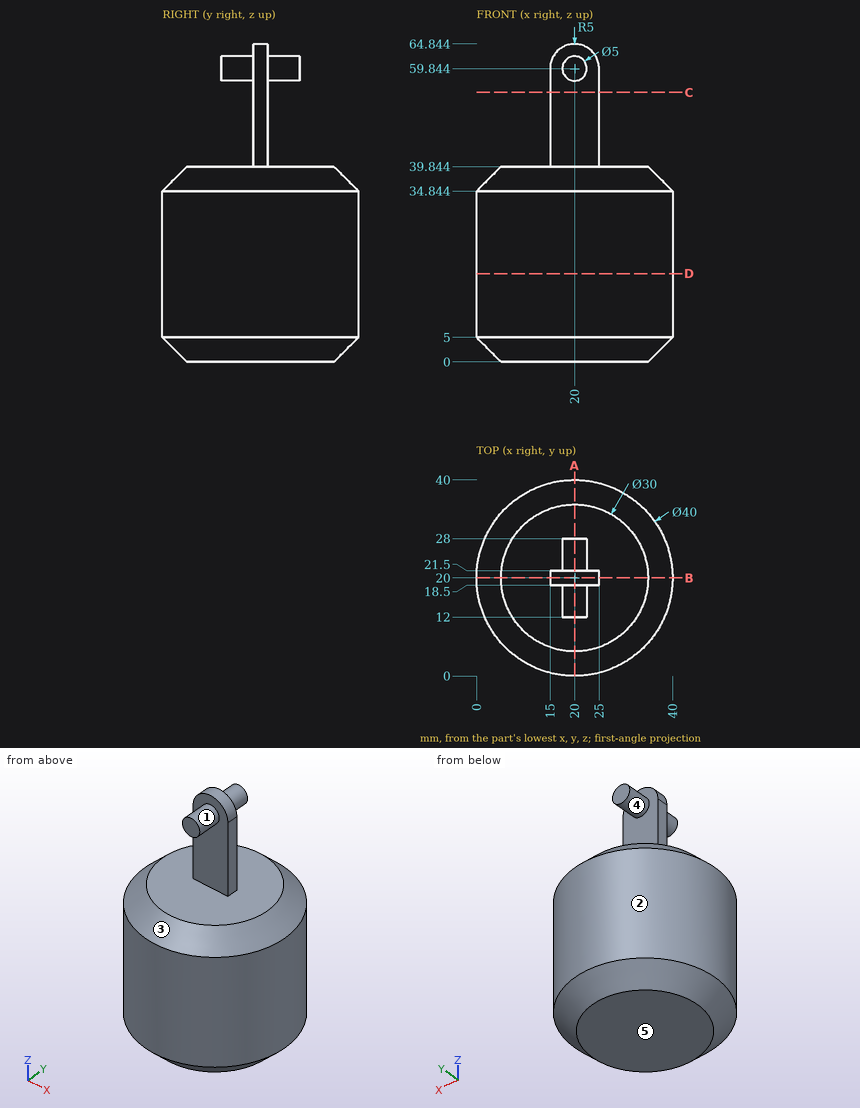
Study the drawing (mm; zero at the part's minimum x, y, z) and answer. A direction names the side the tool comes from. Give positions to 0.01 mm unless a question says otherwise; leave off trailing zeros. Write each loop counter-clockwise with the first axis right and the second up, starting at its lowest first coordinate (ties: lowest second). Pieces come first, ordered by that corner, then holes. Notation, with made-up numbers: M -17,49 L 33,49 A15 ccw 33,71 Z; hole C 48,-26.75 d4. An arc over 180 degrees is marked long. Put each result on its own line as item: value. Start each with the question number.
1. For a pull along Z with two mould halves and no side action, classify the marked faces 1, 2 and 3 as released by +Z, released by -Z, zero draft, split by the parting line, or undercut.
2. Which of the six approach directions +Z, -Z, +X, -X, +Y, -Y give full straight-line access (tool end or side, diameter ignored) to the marked faces 4 and 5?
3. The part is cut by section A-A, the plane x = 20. Give the vertices of the cut face in (y, z), and give its area (3 significant figures).
4. The part is cut by section B-B, the plane y = 20. Give the vertices of the cut face in (x, z), and give its area (3 significant figures).
5. Consider line 1 along Z through (x, y) = (13, 19.5); line 2 along X through (y, z) = (7, 35); line 3 along Y through (x, z) = (20.5, 17). Determine where each line is inside the solid, lowest interval first.
6. The part is cut by section C-C, the plane z = 55. Give the vertices of the cut face in (x, y).
7. The part is cut by section D-D, the plane z = 18. Give the vertices of the cut face in (x, y).
8. Each of these flat-tipped pins is pushed along its axis until it touches: pin 1 Ø3 at (x, z) = (24, 14) entering from -Y; pin 2 Ø3 at (y, z) = (19, 42) entering from -X; pin 3 Ø1.5 at (x, z) = (24, 36) entering from -Y; pin 4 Ø1.5 at (x, z) = (26.5, 52) entering from -Y. Where does it stop, or does it pass through?
Final values:
1. face 1: undercut
1. face 2: zero draft
1. face 3: released by +Z
2. face 4: +Y
2. face 5: -Z, +X, -X, +Y, -Y
3. outline: M 0,5 L 5,0 L 35,0 L 40,5 L 40,34.84 L 35,39.84 L 21.5,39.84 L 21.5,57.34 L 28,57.34 L 28,62.34 L 21.5,62.34 L 21.5,64.84 L 18.5,64.84 L 18.5,62.34 L 12,62.34 L 12,57.34 L 18.5,57.34 L 18.5,39.84 L 5,39.84 L 0,34.84 Z
3. area: 1,680 mm²
4. outline: M 0,5 L 5,0 L 35,0 L 40,5 L 40,34.84 L 35,39.84 L 25,39.84 L 25,59.84 A5 ccw 15,59.84 L 15,39.84 L 5,39.84 L 0,34.84 Z
4. area: 1,780 mm²
5. line 1: z = 0 to 39.84
5. line 2: x = 5.01 to 34.99
5. line 3: y = 0.01 to 39.99
6. outline: M 15,18.5 L 25,18.5 L 25,21.5 L 15,21.5 Z
7. outline: C 20,20 d40
8. pin 1: stops at y = 0.16
8. pin 2: stops at x = 15
8. pin 3: stops at y = 0.8
8. pin 4: passes through
